```python
from build123d import *

# Parameters (mm, degrees)
DODANIE_WYCI_GNI_CIE1_DEPTH = 75
ZAOKR_GLENIE1_R             = 25
WYTNIJ_WYCI_GNI_CIE1_DEPTH  = 75
SZKIC6_R                    = 4
WYTNIJ_WYCI_GNI_CIE2_DEPTH  = 15
SZKIC7_W                    = 35
SZKIC7_H                    = 5
DODANIE_WYCI_GNI_CIE2_DEPTH = 15
WYTNIJ_WYCI_GNI_CIE3_DEPTH  = 15


with BuildPart() as part:
    # Szkic1 → Dodanie-wyciągnięcie1 (new body)
    with BuildSketch(Plane.XY):
        Polygon((0, 0), (38.783164401, 0), (38.783164401, 5), (5, 5), (5, 35), (0, 35), align=None)
    extrude(amount=-DODANIE_WYCI_GNI_CIE1_DEPTH)

    # Zaokrąglenie1
    zaokr_glenie1_edges = [part.edges().sort_by_distance(p)[0] for p in [
        (2.5, 35, -75),
    ]]
    fillet(zaokr_glenie1_edges, radius=ZAOKR_GLENIE1_R)

    # Szkic5 → Wytnij-wyciągnięcie1 (cut)
    with BuildSketch(Plane.XZ):
        Polygon((38.783164401, -55), (25, -75), (38.783164401, -75), align=None)
    extrude(amount=-WYTNIJ_WYCI_GNI_CIE1_DEPTH, mode=Mode.SUBTRACT)

    # Szkic6 → Wytnij-wyciągnięcie2 (cut)
    with BuildSketch(Plane(origin=(0, 5, 0), x_dir=(1, 0, 0), z_dir=(0, 1, 0))):
        with Locations(Location((23.783164401, 55, 0), (0, 0, 180))):
            Circle(SZKIC6_R)
        with Locations(Location((23.783164401, 20, 0), (0, 0, 180))):
            Circle(SZKIC6_R)
    extrude(amount=-WYTNIJ_WYCI_GNI_CIE2_DEPTH, mode=Mode.SUBTRACT)

    # Szkic7 → Dodanie-wyciągnięcie2 (add)
    with BuildSketch(Plane(origin=(0, 5, 0), x_dir=(1, 0, 0), z_dir=(0, 1, 0))):
        with Locations((21.283164401, 2.5)):
            Rectangle(SZKIC7_W, SZKIC7_H)
    extrude(amount=DODANIE_WYCI_GNI_CIE2_DEPTH)

    # Szkic8 → Wytnij-wyciągnięcie3 (cut)
    with BuildSketch(Plane(origin=(0, 0, -5), x_dir=(-1, 0, 0), z_dir=(0, 0, -1))):
        Polygon((-38.783164401, 12), (-17.783164401, 20), (-38.783164401, 20), align=None)
    extrude(amount=-WYTNIJ_WYCI_GNI_CIE3_DEPTH, mode=Mode.SUBTRACT)


solid = part.part
```
Geometry: final body of the model. Coordinates: model frame, mm. A direction names the side the tool comes from. Round coordinates to 2 decimals unless told otherwise and drop trailing zeros. Loops run counter-clockwise (first coordinate to the right, second up) from the corner with the lowest first, then second, coordinate; pieces in that order, holes last. Notation, with made-up numbers: (17, 84.25) -> (45, 84.25) arc R21 ccw to (45, 104.25) -> close; hole circle Ø2 at (71.5, 51). An arc over 180 degrees is marked (long way). Use one line per item in the form item = value. Start each with the question number.
1) Section B-B on y = 6. Output: boundary loops of the cut face in (x, z), then the cut area to 3 significant figures.
2) Line query: L1, parallel to X at y = 30.5, z = -40.5; L2, parallel to Z at x = 7.5, y = 15. Output: solid intervals per line, ascending.
3) Section C-C on z = -31. Output: boundary loops of the cut face in (x, y), then the cut area to 3 significant figures.
4) Draft query along Z for faces 4 (the flat face through (22, 5, -40)), 5 (the flat face through (31.99, 2.46, -64.86)), 6 (the cylindrical face through (24.65, 2.535, -58.905)). Return one class per face: released by +Z, released by -Z, zero draft, split by the parting line, or undercut.
5) Section A-A on z = -20. Output: boundary loops of the cut face in (x, y), then the cut area to 3 significant figures.
6) Access query for faces 1 (the flat face through (15, 10, 0)), 2 (the flat face through (11, 20, -3)), 3 (the flat face through (22, 11, -5)). Directions: +Z, -Z, +X, -X, +Y, -Y. A direction counts if a zero-diameter tool reaches every point of the face in a straight line with its end or side. Return the directions, or none.
7) First-contact query: P1, Ø7.5, axis at x = 21.5, y = 11, coming from the -Z side; P2, Ø6, axis at x = 31, z = -32, coming from the +Y side; P3, Ø2.5, axis at x = 14, z = -3.5, coming from the +Y side. Flat tips, straight axial feed; report the tip coordinate or a pass-through.
8) Section D-D on y = 31. Output: boundary loops of the cut face in (x, z).
Response:
q1.outline = (0, -75) -> (5, -75) -> (5, -5) -> (38.78, -5) -> (38.78, 0) -> (0, 0) -> close
q1.area = 544 mm^2
q2.L1 = 0 to 5
q2.L2 = -5 to 0
q3.outline = (0, 0) -> (38.78, 0) -> (38.78, 5) -> (5, 5) -> (5, 35) -> (0, 35) -> close
q3.area = 344 mm^2
q4.face_4 = zero draft
q4.face_5 = released by -Z
q4.face_6 = undercut
q5.outline = (0, 0) -> (19.78, 0) -> (19.78, 5) -> (5, 5) -> (5, 35) -> (0, 35) -> close; (27.78, 0) -> (38.78, 0) -> (38.78, 5) -> (27.78, 5) -> close
q5.area = 304 mm^2
q6.face_1 = +Z, +X, -X, +Y, -Y
q6.face_2 = +Z, -Z, +X, +Y
q6.face_3 = -Z, +X, +Y
q7.P1 = -5
q7.P2 = 5
q7.P3 = 20
q8.outline = (0, -63.56) -> (5, -63.56) -> (5, 0) -> (0, 0) -> close
